Source: CAD feature listing. Evaluate the final solid. Frame: model axes, mm. A direction names the side the tool comes from. Round coordinates to 2 decimals unless told otherwise and drop trailing zeros. Write each loop counter-clockwise with the first axis right and the second up, starting at its lowest first coordinate (ties: lowest second). Pieces come first, ordered by that corner, then holes. Notation, with made-up numbers: M 89,80 L 122,80 A27 ccw 122,101 Z; hole C -24,65.25 d5. An arc over 180 degrees is marked long. Answer in a Markdown table with one row per item. Add a question column.
Item 1: Cut plane C-C on z = -25.5. Return loops of the section in (x, y).
Item 2: Material intervals for probe 1 along Z at (x, y) = (-18.5, 7); probe 2 along Y at (x, z) = (45, 3) (3 decimals); probe 3 along X at (y, z) = (2, -16), sorted ascending.
Item 3: Cut plane D-D on y = 36.5. Return loops of the section in (x, z), and give its area (3 significant figures).
Item 4: Cut plane A-A on z = 0. Return loops of the section in (x, y).
Item 5: Set-up query: faces 1 (the face through (56.69, -4.17, 13.23)), 2 (the face through (8.721, -3.604, 11.446)), 3 (the face through (60.19, -5.99, 19.03)). Return all of +Z, -Z, +X, -X, +Y, -Y with unobstructed straight access to the full face (end or side cutting, diameter ignored); none if empty.
Item 6: Mould query, pull axis Z, two halves, no side actions, for faces 4 (the face through (49.368, 13.277, -2.948)), 5 (the face through (60.09, -8.85, -9.66)), 6 (the face through (61.318, 4, -13)). Classes: released by +Z, released by -Z, zero draft, split by the parting line, or undercut.
Item 7: Cut plane B-B on x = 47.5. Return loops of the section in (y, z), and give its area (3 significant figures).
Item 8: Contact query for flat-ended pins moving along their axis: pin 1 (4 mm diameter, centred on x = -25.5, y = 15.5, fed in from +Z); pin 2 (8 mm diameter, centred on x = 13.5, z = 14, fed in from -Y); pin 3 (5 mm diameter, centred on x = -24, z = -7, fed in from -Y). Output: stop coordinate, or through.
from build123d import *


with BuildPart() as part:
    # Esquisse1 → Révolution1 (revolve)
    with BuildSketch(Plane.XY, mode=Mode.PRIVATE) as r_volution1_sk:
        with BuildLine():
            Line((-42.799561914, 12), (58.818347085, 12))
            Line((58.818347085, 12), (58.818347085, 13.1))
            Line((58.818347085, 13.1), (61.318347085, 13.1))
            Line((61.318347085, 13.1), (61.318347085, 19.95))
            Line((61.318347085, 19.95), (59.085674073, 19.95))
            ThreePointArc((59.085674073, 19.95), (58.476912644, 19.74335334), (58.119748247, 19.208819045))
            Line((58.119748247, 19.208819045), (56.616869713, 13.6))
            Line((56.616869713, 13.6), (42.318347085, 13.6))
            ThreePointArc((42.318347085, 13.6), (-0.835399263, 44.442149004), (-42.799561914, 12))
        make_face()
    revolve(r_volution1_sk.sketch.rotate(Axis((-48.090955631, 0, 0), (1, 0, 0)), 90), axis=Axis((-48.090955631, 0, 0), (1, 0, 0)))  # turned: the seam where the file's is


solid = part.part
Results below:
| question | item | result |
|---|---|---|
| 1 | outline | C 0,0 d72.82 |
| 2 | probe 1 | -39.81 to -9.75, 9.75 to 39.81 |
| 2 | probe 2 | -13.265 to -11.619, 11.619 to 13.265 |
| 2 | probe 3 | -41.42 to 41.42, 57.29 to 61.32 |
| 3 | outline | C 0,0 d50.74 |
| 3 | area | 2,020 mm2 |
| 4 | outline | M -42.8,-12 A44.45 ccw 42.32,-13.6 L 56.62,-13.6 L 58.12,-19.21 A1 ccw 59.09,-19.95 L 61.32,-19.95 L 61.32,-13.1 L 58.82,-13.1 L 58.82,-12 Z; M -42.8,12 L 58.82,12 L 58.82,13.1 L 61.32,13.1 L 61.32,19.95 L 59.09,19.95 A1 ccw 58.12,19.21 L 56.62,13.6 L 42.32,13.6 A44.45 ccw Z |
| 5 | face 1 | none |
| 5 | face 2 | +X, -X |
| 5 | face 3 | +X |
| 6 | face 4 | split by the parting line |
| 6 | face 5 | undercut |
| 6 | face 6 | zero draft |
| 7 | outline | C 0,0 d27.2; hole C 0,0 d24 |
| 7 | area | 129 mm2 |
| 8 | pin 1 | z = 34.65 |
| 8 | pin 2 | y = -41.68 |
| 8 | pin 3 | y = -38.33 |
